Here's how the part is built. I have some questions about the finished solid (model axes, mm). Face numbers are marked on the shaded views. Coordinates: 2 decimals unless noted, no trailing zeros. Write each loop counter-clockwise with the first axis right and the second up, starting at its lowest first coordinate (ties: lowest second). Pieces come first, ordered by that corner, then holes. Notation, with made-up numbers: M 3,45 L 47,45 A22 cw 47,83 Z; hole C 58,88 d10. An arc over 180 degrees is marked long. Use one line per item in the form item = value. Start each with the question number.
1. Please list where these lines run through material, in increasing order: line 1 along Y through (x, z) = (0, -17); line 2 along Y through (x, z) = (0, -2.7); line 3 along Y through (x, z) = (1.75, -14). Write a range as [from, to].
2. I want a section at D-D, the plane y = -4.75. List the corners of the cut face in (x, z) for me.
3. I want a section at C-C, the plane z = -21. List the corners of the cut face in (x, y) for me.
4. I'm going to push flat-ended pins straight in: pin 1 Ø1.5 at (y, z) = (-6.5, -34.5) entering from +X; pin 2 Ø3 at (y, z) = (7, -15) entering from -X; pin 3 Ø2.5 at (x, y) = (0, 9.5) entering from +Z; pin 4 Ø5 at (x, y) = (0, 0) entering from +Z. Where does each tip first touch, or does it pass through?
5. I want a section at B-B, the plane y = 0. List the corners of the cut face in (x, z) for me.
6. I want a section at A-A, the plane x = 0. List the corners of the cut face in (y, z) for me.
7. Thinking about a two-plate mould opening in X: for the marked faces 1, 2 and 3, which applies, released by +X, released by -X, zero draft, split by the parting line, or undercut?
from build123d import *

# Parameters (mm, degrees)
SKETCH_1_R               = 12.2
SKETCH_1_R_2             = 3
EXTRUDE_1_DEPTH          = 43.8
SKETCH_2_R               = 1.5
CUT_EXTRUDE_1_DEPTH      = 5.5
PATTERN_CIRCULAR_2_COUNT = 3


with BuildPart() as part:
    # Sketch 1 → Extrude 1 (new body)
    with BuildSketch(Plane.XY):
        Circle(SKETCH_1_R)
        Circle(SKETCH_1_R_2, mode=Mode.SUBTRACT)
    extrude(amount=-EXTRUDE_1_DEPTH)

    # Sketch 2 → Cut-Extrude 1 (cut)
    with BuildSketch(Plane.XY):
        with Locations((0, 9.5)):
            Circle(SKETCH_2_R)
    cut_extrude_1 = extrude(amount=-CUT_EXTRUDE_1_DEPTH, mode=Mode.SUBTRACT)

    # Pattern Circular 2: Cut-Extrude 1 ×3 about axis
    pattern_circular_2_axis = Axis((0, 0, 0), (0, 0, 1))
    for i in range(1, PATTERN_CIRCULAR_2_COUNT):
        add(cut_extrude_1.rotate(pattern_circular_2_axis, i * 360 / PATTERN_CIRCULAR_2_COUNT), mode=Mode.SUBTRACT)


solid = part.part
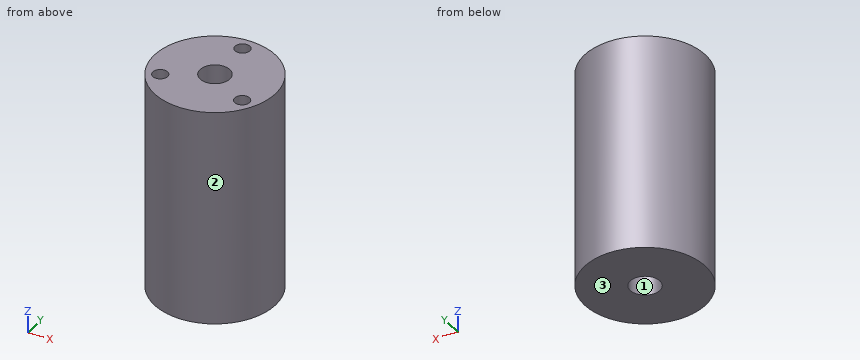
Answer list:
q1.line_1 = [-12.2, -3], [3, 12.2]
q1.line_2 = [-12.2, -3], [3, 8], [11, 12.2]
q1.line_3 = [-12.07, -2.44], [2.44, 12.07]
q2.outline = M -11.24,-43.8 L 11.24,-43.8 L 11.24,0 L 9.73,0 L 9.73,-5.5 L 6.73,-5.5 L 6.73,0 L -6.73,0 L -6.73,-5.5 L -9.73,-5.5 L -9.73,0 L -11.24,0 Z
q3.outline = C 0,0 d24.4; hole C 0,0 d6
q4.pin_1 = 10.76
q4.pin_2 = -10.89
q4.pin_3 = -5.5
q4.pin_4 = through
q5.outline = M -12.2,-43.8 L -3,-43.8 L -3,0 L -12.2,0 Z; M 3,-43.8 L 12.2,-43.8 L 12.2,0 L 3,0 Z
q6.outline = M -12.2,-43.8 L -3,-43.8 L -3,0 L -12.2,0 Z; M 3,-43.8 L 12.2,-43.8 L 12.2,0 L 11,0 L 11,-5.5 L 8,-5.5 L 8,0 L 3,0 Z
q7.face_1 = undercut
q7.face_2 = split by the parting line
q7.face_3 = zero draft
